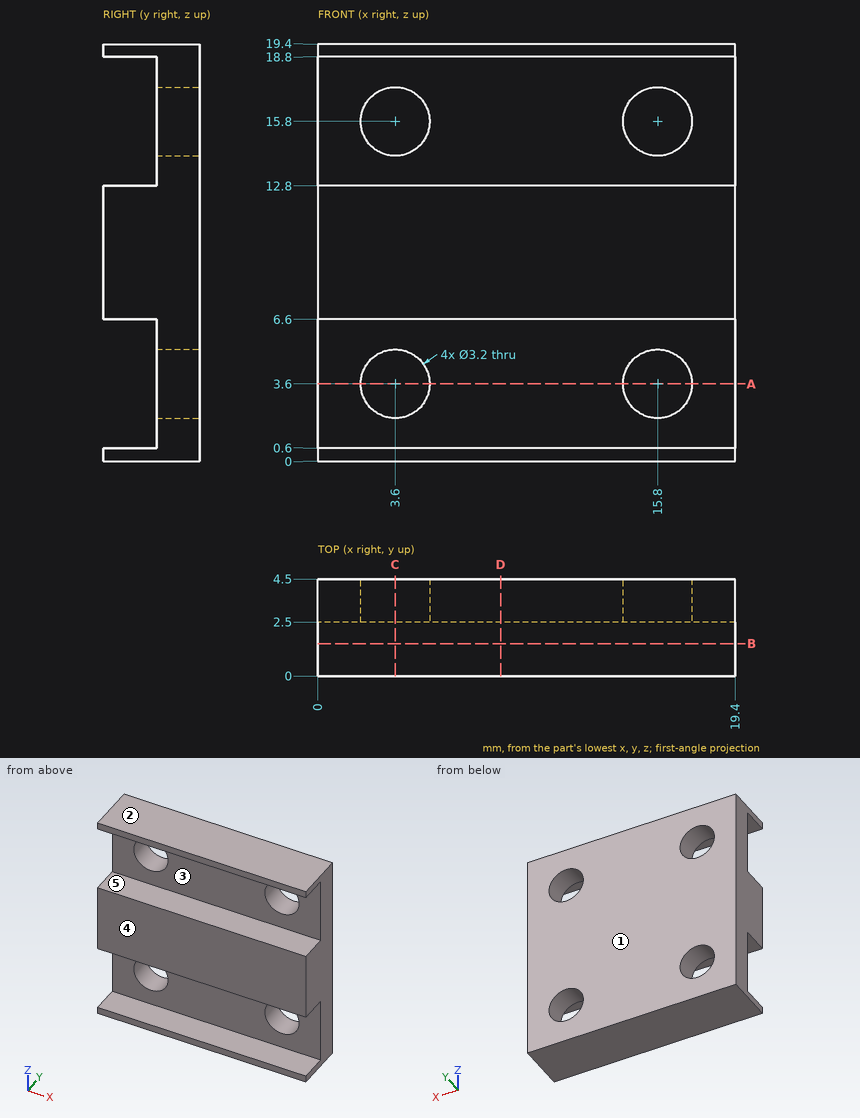
Job drawing, mm, ordinate dimensions from the low corner. One solid piece. A direction names the side the tool comes from. Coordinates: 2 decimals unless noted, no trailing zeros. Order: outer loops, then holes, each group sorted by start corner. A loop starts at its lowest first (then second) coordinate and runs counter-clockwise, first axis right, second up. Notation, with made-up numbers: (72.5, 39) - (113.5, 39) arc R26 cw to (113.5, 77) - close; hole circle Ø1 at (-6.5, 41.25). An arc over 180 degrees is marked (long way). Return JSON: item names as keys, results as strings. Group by question number.
1) Saw through at C-C, the plane x = 3.6. Write the cut outline in (y, z), plus the area to 3 significant figures.
2) Probe line 1 (Z direction, x = 3.6, y = 4.05); line 2 (Z direction, x = 6, y = 0.3). List the from-to ranges inside material, lowest first. Write a range as from..to.
3) Mould opens along Z. For the marked faces 1, 2 and 3 say: released by +Z, released by -Z, zero draft, split by the parting line, or undercut.
4) Saw through at D-D, the plane x = 8.5. Write the cut outline in (y, z).
5) Saw through at B-B, the plane y = 1.5. Write the cut outline in (x, z).
6) Tool access for the marked faces 4 and 5: list every direction of +Z, -Z, +X, -X, +Y, -Y with a clear straight run to the whole face (end or side of a thin tool).
7) Saw through at A-A, the plane z = 3.6. Write the cut outline in (x, y), plus the area to 3 significant figures.
8) Flat gauge pin, fed straight in: P1, Ø3.5, axis at x = 15.8, z = 3.6, coming from the -Y side. Where does the tip first touch, or does it go through?
Values found:
{
 "1": {"outline": "(0, 0) - (4.5, 0) - (4.5, 2) - (2.5, 2) - (2.5, 0.6) - (0, 0.6) - close; (0, 6.6) - (2.5, 6.6) - (2.5, 5.2) - (4.5, 5.2) - (4.5, 14.2) - (2.5, 14.2) - (2.5, 12.8) - (0, 12.8) - close; (0, 18.8) - (2.5, 18.8) - (2.5, 17.4) - (4.5, 17.4) - (4.5, 19.4) - (0, 19.4) - close", "area": "44.5 mm²"},
 "2": {"line 1": "z = 0..2, 5.2..14.2, 17.4..19.4", "line 2": "z = 0..0.6, 6.6..12.8, 18.8..19.4"},
 "3": {"face 1": "zero draft", "face 2": "released by +Z", "face 3": "undercut"},
 "4": {"outline": "(0, 0) - (4.5, 0) - (4.5, 19.4) - (0, 19.4) - (0, 18.8) - (2.5, 18.8) - (2.5, 12.8) - (0, 12.8) - (0, 6.6) - (2.5, 6.6) - (2.5, 0.6) - (0, 0.6) - close"},
 "5": {"outline": "(0, 0) - (19.4, 0) - (19.4, 0.6) - (0, 0.6) - close; (0, 6.6) - (19.4, 6.6) - (19.4, 12.8) - (0, 12.8) - close; (0, 18.8) - (19.4, 18.8) - (19.4, 19.4) - (0, 19.4) - close"},
 "6": {"face 4": "+Z, -Z, +X, -X, -Y", "face 5": "+X, -X, -Y"},
 "7": {"outline": "(0, 2.5) - (2, 2.5) - (2, 4.5) - (0, 4.5) - close; (5.2, 2.5) - (14.2, 2.5) - (14.2, 4.5) - (5.2, 4.5) - close; (17.4, 2.5) - (19.4, 2.5) - (19.4, 4.5) - (17.4, 4.5) - close", "area": "26.0 mm²"},
 "8": {"P1": "stops at y = 2.5"}
}
